```python
from build123d import *

# Parameters (mm, degrees)
SKETCH1_W                = 152.4
SKETCH1_H                = 38.1
BOSS_EXTRUDE1_DEPTH      = 6.35
SKETCH2_R                = 3.175
CUT_EXTRUDE1_DEPTH       = 7.35
SKETCH3_W                = 152.4
SKETCH3_H                = 12.7
BOSS_EXTRUDE2_DEPTH      = 139.7
SKETCH4_W                = 82.55
SKETCH4_H                = 12.793482267
BOSS_EXTRUDE3_DEPTH      = 88.9
BOSS_EXTRUDE3_DEPTH_BACK = 152.4
SKETCH5_W                = 88.9
SKETCH5_H                = 44.45
CUT_EXTRUDE2_DEPTH       = 152.4
CUT_EXTRUDE3_DEPTH       = 242.3
BOSS_EXTRUDE4_DEPTH      = 241.3


with BuildPart() as part:
    # Sketch1 → Boss-Extrude1 (new body)
    with BuildSketch(Plane(origin=(0, 0, 0), x_dir=(1, 0, 0), z_dir=(0, 1, 0))):
        with Locations((69.256115108, 12.928417266)):
            Rectangle(SKETCH1_W, SKETCH1_H)
    extrude(amount=BOSS_EXTRUDE1_DEPTH)

    # Sketch2 → Cut-Extrude1 (cut, through all)
    with BuildSketch(Plane(origin=(0, 6.35, 0), x_dir=(1, 0, 0), z_dir=(0, 1, 0))):
        with Locations((-0.593884892, 12.928417266)):
            Circle(SKETCH2_R)
        with Locations((24.806115108, 12.928417266)):
            Circle(SKETCH2_R)
        with Locations((50.206115108, 12.928417266)):
            Circle(SKETCH2_R)
        with Locations((75.606115108, 12.928417266)):
            Circle(SKETCH2_R)
        with Locations((101.006115108, 12.928417266)):
            Circle(SKETCH2_R)
        with Locations((126.406115108, 12.928417266)):
            Circle(SKETCH2_R)
    extrude(amount=-CUT_EXTRUDE1_DEPTH, mode=Mode.SUBTRACT)

    # Sketch3 → Boss-Extrude2 (add)
    with BuildSketch(Plane(origin=(0, 6.35, 0), x_dir=(1, 0, 0), z_dir=(0, 1, 0))):
        with Locations((69.256115108, 0.228417266)):
            Rectangle(SKETCH3_W, SKETCH3_H)
    extrude(amount=BOSS_EXTRUDE2_DEPTH)

    # Sketch4 → Boss-Extrude3 (add, two sides)
    with BuildSketch(Plane.ZY.offset(6.943884892)) as boss_extrude3_sk:
        with Locations((34.696582734, 139.653258867)):
            Rectangle(SKETCH4_W, SKETCH4_H)
    extrude(amount=BOSS_EXTRUDE3_DEPTH)
    extrude(boss_extrude3_sk.sketch, amount=-BOSS_EXTRUDE3_DEPTH_BACK)

    # Sketch5 → Cut-Extrude2 (cut)
    with BuildSketch(Plane(origin=(0, 146.05, 0), x_dir=(1, 0, 0), z_dir=(0, 1, 0))):
        with Locations((-51.393884892, -15.646582734)):
            Rectangle(SKETCH5_W, SKETCH5_H)
    extrude(amount=-CUT_EXTRUDE2_DEPTH, mode=Mode.SUBTRACT)

    # Sketch6 → Cut-Extrude3 (cut, through all)
    with BuildSketch(Plane.ZY.offset(95.843884892)):
        Polygon((75.971582734, 146.05), (63.178100467, 133.256517733), (75.971582734, 133.256517733), align=None)
    extrude(amount=-CUT_EXTRUDE3_DEPTH, mode=Mode.SUBTRACT)

    # Sketch7 → Boss-Extrude4 (add, through all)
    with BuildSketch(Plane.ZY.offset(95.843884892)):
        Polygon((84.951838855, 155.030256121), (83.155787631, 156.826307345), (65.195275389, 138.865795103), (66.991326613, 137.069743879), align=None)
    extrude(amount=-BOSS_EXTRUDE4_DEPTH)


solid = part.part
```
For this review, take the finished solid that the model builds, in its own axes (mm). A direction names the side the tool comes from. Round coordinates to 2 decimals unless told otherwise and drop trailing zeros. Write each loop counter-clockwise with the first axis right and the second up, starting at its lowest first coordinate (ties: lowest second). Pieces come first, ordered by that corner, then holes. Notation, with made-up numbers: (80.25, -6.75) -> (118.25, -6.75) arc R22 ccw to (118.25, 31.25) -> close; hole circle Ø4 at (7.5, 88). An arc over 180 degrees is marked (long way). Use one line per item in the form item = value.
Q1. Consider section D-D (x = 100.5). State the section outline as (y, z) points, then the cut area to 3 significant figures.
Resolved:
outline = (0, -31.98) -> (6.35, -31.98) -> (6.35, -16.06) -> (0, -16.06) -> close; (0, -9.79) -> (6.35, -9.79) -> (6.35, -6.58) -> (146.05, -6.58) -> (146.05, 72.38) -> (156.83, 83.16) -> (155.03, 84.95) -> (133.26, 63.18) -> (133.26, 6.12) -> (0, 6.12) -> close
area = 2,820 mm²
Q2. Clearance check with flat-ended pins moving along their axes: pin 1 Ø4 at (x, y) = (28.5, 126.5) entering from +Z; pin 2 Ø3 at (x, z) = (117.5, 53.5) entering from -Y; pin 3 Ø4 at (x, z) = (126.41, -12.93) entering from -Y; pin 4 Ø7.5 at (x, z) = (38.5, -24) entering from +Y. State where each tip first meets the part, or that it passes through.
Resolved:
pin_1 = 6.12
pin_2 = 133.26
pin_3 = through
pin_4 = 6.35
Q3. Consider section B-B (y = 98). State the section outline as (x, z) points, then the cut area to 3 significant figures.
Resolved:
outline = (-6.94, -6.58) -> (145.46, -6.58) -> (145.46, 6.12) -> (-6.94, 6.12) -> close
area = 1,940 mm²
Q4. The part is to be moulded in two halves that separate along Z. For faces 4 (the flat face through (68, 66, 6.122)), 5 (the flat face through (53, 133.257, 34)), 6 (the flat face through (23.12, 151.51, 77.84)), 7 (the cylindrical face through (104.034, 3.219, -13.882)), say which applies: released by +Z, released by -Z, zero draft, split by the parting line, or undercut.
Resolved:
face_4 = released by +Z
face_5 = zero draft
face_6 = released by -Z
face_7 = undercut
Q5. Machinability: for faces 1 (the flat face through (-52, 140, 37.872)), 2 (the flat face through (70, 75, -6.578)), 3 (the flat face through (-95.844, 140, 56)), which of the approach directions +Z, -Z, +X, -X, +Y, -Y give a long, thin tool a straight path to every point of the face, cutting with its end or side? Answer none if there is none.
Resolved:
face_1 = -Z, -X, +Y, -Y
face_2 = -Z, +X, -X, +Y
face_3 = +Z, -Z, -X, +Y, -Y
Q6. To check wall thickness, follow probe 1 along Y at (x, z) = (14, 60); probe 2 along Z at (x, y) = (126, 50); probe 3 along Y at (x, z) = (29.5, 0). State the ranges of each line that lie inside material, in increasing order. Write a range as from..to.
Resolved:
probe_1 = 133.26..146.05
probe_2 = -6.58..6.12
probe_3 = 0..146.05
Q7. Consider section C-C (z = 58.5). State the section outline as (x, y) points.
Resolved:
outline = (-95.84, 133.26) -> (145.46, 133.26) -> (145.46, 146.05) -> (-95.84, 146.05) -> close
Q8. Consider section A-A (x = 43.5). State the section outline as (y, z) points, then the cut area to 3 significant figures.
Resolved:
outline = (0, -31.98) -> (6.35, -31.98) -> (6.35, -6.58) -> (146.05, -6.58) -> (146.05, 72.38) -> (156.83, 83.16) -> (155.03, 84.95) -> (133.26, 63.18) -> (133.26, 6.12) -> (0, 6.12) -> close
area = 2,860 mm²
